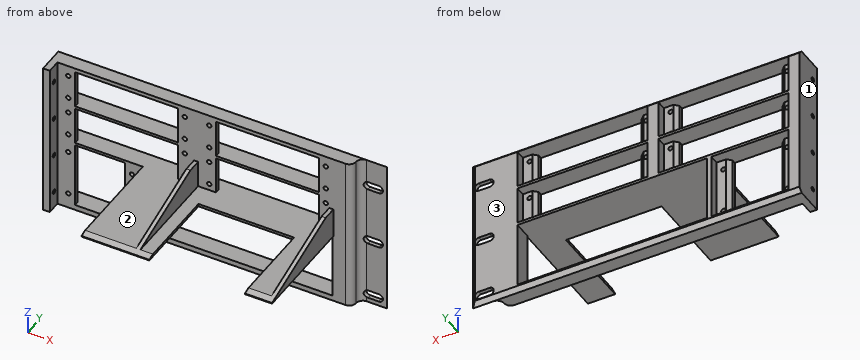
```python
from build123d import *

# Parameters (mm, degrees)
SKETCH1_W                      = 242.5
SKETCH1_H                      = 116
BOSS_EXTRUDE1_DEPTH            = 13
SKETCH32_W                     = 20
SKETCH32_H                     = 116
CUT_EXTRUDE10_DEPTH            = 10
FILLET1_START                  = -59
FILLET1_DEPTH                  = 118
FILLET1_START_2                = -58
FILLET1_2_DEPTH                = 116
SKETCH36_W                     = 96
SKETCH36_H                     = 28
CUT_EXTRUDE11_DEPTH            = 7
SKETCH37_W                     = 76
SKETCH37_H                     = 28
CUT_EXTRUDE12_DEPTH            = 143.489473295
M4X0_7_TAPPED_HOLE1_AT_2_COUNT = 2
M4X0_7_TAPPED_HOLE1_AT_2_PITCH = 18
M4X0_7_TAPPED_HOLE1_AT_3_COUNT = 2
M4X0_7_TAPPED_HOLE1_AT_3_PITCH = 86
M4X0_7_TAPPED_HOLE1_AT_4_COUNT = 2
M4X0_7_TAPPED_HOLE1_AT_4_PITCH = 87.863530546
LPATTERN1_COUNT                = 2
LPATTERN1_PITCH                = 30
LPATTERN1_COUNT_DIR2           = 2
LPATTERN1_PITCH_DIR2           = 104
CHAMFER1_SIZE                  = 3
SKETCH41_W                     = 140
SKETCH41_H                     = 49
CUT_EXTRUDE13_DEPTH            = 30
BOSS_EXTRUDE2_DEPTH            = 80
SKETCH43_W                     = 57
SKETCH43_H                     = 49
CUT_EXTRUDE14_DEPTH            = 7
SKETCH44_W                     = 37
SKETCH44_H                     = 49
CUT_EXTRUDE15_DEPTH            = 17
CHAMFER2_SIZE                  = 3
M4X0_7_TAPPED_HOLE2_D          = 3.3
M4X0_7_TAPPED_HOLE2_DEPTH      = 10.1
M4X0_7_TAPPED_HOLE2_TIP        = 0.991420021
CHAMFER3_SIZE                  = 70
CHAMFER3_SIZE2                 = 21.401147702
SKETCH48_W                     = 5
SKETCH48_H                     = 116
BOSS_EXTRUDE3_DEPTH            = 10
SKETCH49_W                     = 70.567921878
SKETCH49_H                     = 64.139989259
CUT_EXTRUDE16_DEPTH            = 10
M4X0_7_TAPPED_HOLE3_D          = 3.3
M4X0_7_TAPPED_HOLE3_DEPTH      = 5
CUT_EXTRUDE17_DEPTH            = 170.656270146


with BuildPart() as part:
    # Sketch1 → Boss-Extrude1 (new body)
    with BuildSketch(Plane(origin=(0, 0, 0), x_dir=(1, 0, 0), z_dir=(0, 1, 0))):
        with Locations((8.25, 0)):
            Rectangle(SKETCH1_W, SKETCH1_H)
    extrude(amount=BOSS_EXTRUDE1_DEPTH)

    # Sketch32 → Cut-Extrude10 (cut)
    with BuildSketch(Plane.XZ):
        with Locations((119.5, 0)):
            Rectangle(SKETCH32_W, SKETCH32_H)
    extrude(amount=-CUT_EXTRUDE10_DEPTH, mode=Mode.SUBTRACT)

    # Fillet1: read off the stored shape, not the designer's step
    # Fillet1 outline → Fillet1 (cut)
    with BuildSketch(Plane.XY.offset(FILLET1_START)):
        with BuildLine():
            Line((109.5, 0), (109.5, 5))
            ThreePointArc((109.5, 5), (108.035533906, 1.464466094), (104.5, 0))
            Line((104.5, 0), (109.5, 0))
        make_face()
    extrude(amount=FILLET1_DEPTH, mode=Mode.SUBTRACT)

    # Fillet1 2 outline → Fillet1 2 (add)
    with BuildSketch(Plane.XY.offset(FILLET1_START_2)):
        with BuildLine():
            ThreePointArc((109.5, 5), (110.964466094, 8.535533906), (114.5, 10))
            Line((114.5, 10), (109.5, 10))
            Line((109.5, 10), (109.5, 5))
        make_face()
    extrude(amount=FILLET1_2_DEPTH)

    # Sketch36 → Cut-Extrude11 (cut)
    with BuildSketch(Plane(origin=(0, 13, 0), x_dir=(1, 0, 0), z_dir=(0, 1, 0))):
        with Locations((-57, -41)):
            Rectangle(SKETCH36_W, SKETCH36_H)
        with Locations((-57, -11)):
            Rectangle(SKETCH36_W, SKETCH36_H)
        with Locations((47, -11)):
            Rectangle(SKETCH36_W, SKETCH36_H)
        with Locations((47, -41)):
            Rectangle(SKETCH36_W, SKETCH36_H)
    extrude(amount=-CUT_EXTRUDE11_DEPTH, mode=Mode.SUBTRACT)

    # Sketch37 → Cut-Extrude12 (cut, through all)
    with BuildSketch(Plane(origin=(0, 13, 0), x_dir=(1, 0, 0), z_dir=(0, 1, 0))):
        with Locations((-57, -41)):
            Rectangle(SKETCH37_W, SKETCH37_H)
        with Locations((-57, -11)):
            Rectangle(SKETCH37_W, SKETCH37_H)
        with Locations((47, -11)):
            Rectangle(SKETCH37_W, SKETCH37_H)
        with Locations((47, -41)):
            Rectangle(SKETCH37_W, SKETCH37_H)
    extrude(amount=-CUT_EXTRUDE12_DEPTH, mode=Mode.SUBTRACT)

    # Sketch39 → M4x0.7 Tapped Hole1 (revolve, cut)
    with BuildSketch(Plane(origin=(-100, 6, 50), x_dir=(0, 0, 1), z_dir=(1, 0, 0))):
        Polygon((0, 0), (0, 11.091420021), (1.65, 10.1), (1.65, 0), align=None)
    m4x0_7_tapped_hole1 = revolve(axis=Axis((-100, 12.35, 50), (0, -1, 0)), mode=Mode.SUBTRACT)

    # M4x0.7 Tapped Hole1 at 2: M4x0.7 Tapped Hole1 ×2
    with Locations(*[(0, 0, -i * M4X0_7_TAPPED_HOLE1_AT_2_PITCH) for i in range(1, M4X0_7_TAPPED_HOLE1_AT_2_COUNT)]):
        add(m4x0_7_tapped_hole1, mode=Mode.SUBTRACT)

    # M4x0.7 Tapped Hole1 at 3: M4x0.7 Tapped Hole1 ×2
    with Locations(*[(i * M4X0_7_TAPPED_HOLE1_AT_3_PITCH, 0, 0) for i in range(1, M4X0_7_TAPPED_HOLE1_AT_3_COUNT)]):
        add(m4x0_7_tapped_hole1, mode=Mode.SUBTRACT)

    # M4x0.7 Tapped Hole1 at 4: M4x0.7 Tapped Hole1 ×2
    with Locations(*[Vector(0.9787906252528686, 0, -0.20486315412269346) * (i * M4X0_7_TAPPED_HOLE1_AT_4_PITCH) for i in range(1, M4X0_7_TAPPED_HOLE1_AT_4_COUNT)]):
        add(m4x0_7_tapped_hole1, mode=Mode.SUBTRACT)

    # LPattern1: M4x0.7 Tapped Hole1 2 × 2
    with Locations(*[(j * LPATTERN1_PITCH_DIR2, 0, -i * LPATTERN1_PITCH) for i in range(LPATTERN1_COUNT) for j in range(LPATTERN1_COUNT_DIR2) if (i, j) != (0, 0)]):
        add(m4x0_7_tapped_hole1, mode=Mode.SUBTRACT)

    # LPattern1 copy 1 sketch → LPattern1 copy 1 (revolve, cut)
    with BuildSketch(Plane(origin=(4, 6, 32), x_dir=(0, 0, 1), z_dir=(1, 0, 0))):
        Polygon((0, 0), (0, 11.091420021), (1.65, 10.1), (1.65, 0), align=None)
    revolve(axis=Axis((4, 12.35, 32), (0, -1, 0)), mode=Mode.SUBTRACT)

    # LPattern1 copy 2 sketch → LPattern1 copy 2 (revolve, cut)
    with BuildSketch(Plane(origin=(-100, 6, 2), x_dir=(0, 0, 1), z_dir=(1, 0, 0))):
        Polygon((0, 0), (0, 11.091420021), (1.65, 10.1), (1.65, 0), align=None)
    revolve(axis=Axis((-100, 12.35, 2), (0, -1, 0)), mode=Mode.SUBTRACT)

    # LPattern1 copy 3 sketch → LPattern1 copy 3 (revolve, cut)
    with BuildSketch(Plane(origin=(4, 6, 2), x_dir=(0, 0, 1), z_dir=(1, 0, 0))):
        Polygon((0, 0), (0, 11.091420021), (1.65, 10.1), (1.65, 0), align=None)
    revolve(axis=Axis((4, 12.35, 2), (0, -1, 0)), mode=Mode.SUBTRACT)

    # LPattern1 copy 4 sketch → LPattern1 copy 4 (revolve, cut)
    with BuildSketch(Plane(origin=(90, 6, 50), x_dir=(0, 0, 1), z_dir=(1, 0, 0))):
        Polygon((0, 0), (0, 11.091420021), (1.65, 10.1), (1.65, 0), align=None)
    revolve(axis=Axis((90, 12.35, 50), (0, -1, 0)), mode=Mode.SUBTRACT)

    # LPattern1 copy 5 sketch → LPattern1 copy 5 (revolve, cut)
    with BuildSketch(Plane(origin=(-14, 6, 20), x_dir=(0, 0, 1), z_dir=(1, 0, 0))):
        Polygon((0, 0), (0, 11.091420021), (1.65, 10.1), (1.65, 0), align=None)
    revolve(axis=Axis((-14, 12.35, 20), (0, -1, 0)), mode=Mode.SUBTRACT)

    # LPattern1 copy 6 sketch → LPattern1 copy 6 (revolve, cut)
    with BuildSketch(Plane(origin=(90, 6, 20), x_dir=(0, 0, 1), z_dir=(1, 0, 0))):
        Polygon((0, 0), (0, 11.091420021), (1.65, 10.1), (1.65, 0), align=None)
    revolve(axis=Axis((90, 12.35, 20), (0, -1, 0)), mode=Mode.SUBTRACT)

    # LPattern1 copy 7 sketch → LPattern1 copy 7 (revolve, cut)
    with BuildSketch(Plane(origin=(90, 6, 32), x_dir=(0, 0, 1), z_dir=(1, 0, 0))):
        Polygon((0, 0), (0, 11.091420021), (1.65, 10.1), (1.65, 0), align=None)
    revolve(axis=Axis((90, 12.35, 32), (0, -1, 0)), mode=Mode.SUBTRACT)

    # LPattern1 copy 8 sketch → LPattern1 copy 8 (revolve, cut)
    with BuildSketch(Plane(origin=(-14, 6, 2), x_dir=(0, 0, 1), z_dir=(1, 0, 0))):
        Polygon((0, 0), (0, 11.091420021), (1.65, 10.1), (1.65, 0), align=None)
    revolve(axis=Axis((-14, 12.35, 2), (0, -1, 0)), mode=Mode.SUBTRACT)

    # LPattern1 copy 9 sketch → LPattern1 copy 9 (revolve, cut)
    with BuildSketch(Plane(origin=(90, 6, 2), x_dir=(0, 0, 1), z_dir=(1, 0, 0))):
        Polygon((0, 0), (0, 11.091420021), (1.65, 10.1), (1.65, 0), align=None)
    revolve(axis=Axis((90, 12.35, 2), (0, -1, 0)), mode=Mode.SUBTRACT)

    # Chamfer1
    chamfer1_edges = [part.edges().sort_by_distance(p)[0] for p in [
        (-95, 6, 11),
        (-19, 6, 11),
        (-19, 6, 41),
        (-95, 6, 41),
        (85, 6, 11),
        (9, 6, 11),
        (9, 6, 41),
        (85, 6, 41),
        (8.25, 13, -58),
        (129.5, 13, 0),
        (8.25, 13, 58),
    ]]
    chamfer(chamfer1_edges, length=CHAMFER1_SIZE - 0.0001)  # a hair under: the kernel refuses the full size

    # Sketch41 → Cut-Extrude13 (cut)
    with BuildSketch(Plane(origin=(0, 13, 0), x_dir=(1, 0, 0), z_dir=(0, 1, 0))):
        with Locations((25, 29.5)):
            Rectangle(SKETCH41_W, SKETCH41_H)
    extrude(amount=-CUT_EXTRUDE13_DEPTH, mode=Mode.SUBTRACT)

    # Sketch42 → Boss-Extrude2 (add)
    with BuildSketch(Plane.XZ):
        Polygon((-45, -5), (-45, -3), (-7.207942419, -3), (-7.207942419, 16.976819085), (-4.207942419, 16.976819085), (-4.207942419, -3), (92.567921878, -3), (92.567921878, 16.976819085), (95.567921878, 16.976819085), (95.567921878, -5), align=None)
    extrude(amount=BOSS_EXTRUDE2_DEPTH)

    # Sketch43 → Cut-Extrude14 (cut)
    with BuildSketch(Plane(origin=(0, 13, 0), x_dir=(1, 0, 0), z_dir=(0, 1, 0))):
        with Locations((-76.5, 29.5)):
            Rectangle(SKETCH43_W, SKETCH43_H)
    extrude(amount=-CUT_EXTRUDE14_DEPTH, mode=Mode.SUBTRACT)

    # Sketch44 → Cut-Extrude15 (cut)
    with BuildSketch(Plane(origin=(0, 6, 0), x_dir=(1, 0, 0), z_dir=(0, 1, 0))):
        with Locations((-76.5, 29.5)):
            Rectangle(SKETCH44_W, SKETCH44_H)
    extrude(amount=-CUT_EXTRUDE15_DEPTH, mode=Mode.SUBTRACT)

    # Chamfer2
    chamfer2_edges = [part.edges().sort_by_distance(p)[0] for p in [
        (-95, 6, -29.5),
        (-58, 6, -29.5),
    ]]
    chamfer(chamfer2_edges, length=CHAMFER2_SIZE)

    # M4x0.7 Tapped Hole2
    with Locations(Plane(origin=(0, 6, 0), x_dir=(1, 0, 0), z_dir=(0, 1, 0))):
        with Locations((-100, 12.5), (-100, 46.5), (-53, 46.5), (-53, 12.5)):
            Hole(M4X0_7_TAPPED_HOLE2_D / 2, depth=M4X0_7_TAPPED_HOLE2_DEPTH)
            with Locations((0, 0, -(M4X0_7_TAPPED_HOLE2_DEPTH + M4X0_7_TAPPED_HOLE2_TIP / 2))):  # 118° drill point
                Cone(0, M4X0_7_TAPPED_HOLE2_D / 2, M4X0_7_TAPPED_HOLE2_TIP, mode=Mode.SUBTRACT)

    # Chamfer3
    chamfer3_edges = [part.edges().sort_by_distance(p)[0] for p in [
        (-5.707942419, -80, 16.976819085),
    ]]
    chamfer3_side = [part.faces().sort_by_distance(p)[0] for p in [
        (-5.707942419, -40, 16.976819085),
    ]]
    chamfer(chamfer3_edges, length=CHAMFER3_SIZE, length2=CHAMFER3_SIZE2, reference=chamfer3_side[0])

    # Sketch48 → Boss-Extrude3 (add)
    with BuildSketch(Plane.XZ):
        with Locations((-110.5, 0)):
            Rectangle(SKETCH48_W, SKETCH48_H)
    extrude(amount=BOSS_EXTRUDE3_DEPTH)

    # Sketch49 → Cut-Extrude16 (cut)
    with BuildSketch(Plane(origin=(0, 0, -5), x_dir=(-1, 0, 0), z_dir=(0, 0, -1))):
        with Locations((-40.283960939, -47.93000537)):
            Rectangle(SKETCH49_W, SKETCH49_H)
    extrude(amount=-CUT_EXTRUDE16_DEPTH, mode=Mode.SUBTRACT)

    # M4x0.7 Tapped Hole3
    with Locations(Plane(origin=(-108, 0, 0), x_dir=(0, 0, -1), z_dir=(1, 0, 0))):
        with Locations((15, -4.5), (45, -4.5), (-15, -4.5), (-45, -4.5)):
            Hole(M4X0_7_TAPPED_HOLE3_D / 2, depth=M4X0_7_TAPPED_HOLE3_DEPTH)

    # Sketch53 → Cut-Extrude17 (cut, through all)
    with BuildSketch(Plane(origin=(0, 13, 0), x_dir=(1, 0, 0), z_dir=(0, 1, 0))):
        with BuildLine():
            Line((123.5, 48.65), (115.5, 48.65))
            ThreePointArc((115.5, 48.65), (112.5, 51.65), (115.5, 54.65))
            Line((115.5, 54.65), (123.5, 54.65))
            ThreePointArc((123.5, 54.65), (126.5, 51.65), (123.5, 48.65))
        make_face()
        with BuildLine():
            Line((123.5, 4.2), (115.5, 4.2))
            ThreePointArc((115.5, 4.2), (112.5, 7.2), (115.5, 10.2))
            Line((115.5, 10.2), (123.5, 10.2))
            ThreePointArc((123.5, 10.2), (126.5, 7.2), (123.5, 4.2))
        make_face()
        with BuildLine():
            Line((123.5, -40.25), (115.5, -40.25))
            ThreePointArc((115.5, -40.25), (112.5, -37.25), (115.5, -34.25))
            Line((115.5, -34.25), (123.5, -34.25))
            ThreePointArc((123.5, -34.25), (126.5, -37.25), (123.5, -40.25))
        make_face()
    extrude(amount=-CUT_EXTRUDE17_DEPTH, mode=Mode.SUBTRACT)


solid = part.part
```
Work out the finished part from the listing and answer in its coordinate system (mm). Face numbers are marked on the shaded views. Give positions to 0.01 mm unless a question says otherwise; leave off trailing zeros. Order: outer loops, then holes, each group sorted by start corner. A loop starts at its lowest first (then second) coordinate and runs counter-clockwise, first axis right, second up. Notation, with made-up numbers: (-25, 62) - (1, 62) arc R20 cw to (1, 75) - close; hole circle Ø3 at (13, -8.75). An arc over 180 degrees is marked (long way). One line per item, written item: value. Start each with the question number.
1. Each of these flat-tipped pins is pushed along its axis until it touches: pin 1 Ø4 at (x, z) = (-100, -12.5) entering from +Y; pin 2 Ø3 at (y, z) = (-7, -22) entering from +X; pin 3 Ø0.9 at (y, z) = (2, 44) entering from +X; pin 4 Ø2 at (x, z) = (4, 2) entering from +Y. Where does it stop, or does it pass through?
2. Section C-C, the plane y = -26.5 is taken. Write down the section's boundary in (x, z), then the cut area to 3 significant figures.
3. Consider line 1 (X direction, y = -8, z = 9.5); line 2 (X direction, y = 4.3, z = -12.5); line 3 (Y direction, x = -109.4, z = -15). Determine where each line is inside the solid, lowest interval first.
4. Section D-D, the plane y = -67.5 is taken. Write down the section's boundary in (x, z), then the cut area to 3 significant figures.
5. For a pull along X with two mould halves and no side action, classify the marked faces 1, 2 and 3 as released by +X, released by -X, zero draft, split by the parting line, or undercut.
6. Section A-A, the plane z = -26.5 is taken. Count the separate pieces of the cut face and the enclosed holes in it, then the cut area to 3 significant figures.
Filled sheet:
1. pin 1: y = 6
1. pin 2: x = -108
1. pin 3: x = 108.8
1. pin 4: through
2. outline: (-45, -5) - (5, -5) - (5, -3) - (-4.21, -3) - (-4.21, 11.93) - (-7.21, 11.93) - (-7.21, -3) - (-45, -3) - close; (75.57, -5) - (95.57, -5) - (95.57, 11.93) - (92.57, 11.93) - (92.57, -3) - (75.57, -3) - close
2. area: 230 mm²
3. line 1: -113 to -108, -7.21 to -4.21, 92.57 to 95.57
3. line 2: -113 to -101.65, -98.35 to -96.3, -56.7 to -54.65, -51.35 to -45, 95 to 109.45
3. line 3: -10 to -6.15, -2.85 to 13
4. outline: (-45, -5) - (5, -5) - (5, -3) - (-4.21, -3) - (-4.21, -0.6) - (-7.21, -0.6) - (-7.21, -3) - (-45, -3) - close; (75.57, -5) - (95.57, -5) - (95.57, -0.6) - (92.57, -0.6) - (92.57, -3) - (75.57, -3) - close
4. area: 154 mm²
5. face 1: released by -X
5. face 2: undercut
5. face 3: zero draft
6. separate pieces: 3
6. enclosed holes: 0
6. area: 548 mm²
